from build123d import *

# Parameters (mm, degrees)
CORTAR_EXTRUIR1_DEPTH   = 9
CROQUIS5_R              = 4
CORTAR_EXTRUIR3_DEPTH   = 27
CROQUIS6_R              = 2
CORTAR_EXTRUIR4_DEPTH   = 10
CROQUIS7_R              = 2
SALIENTE_EXTRUIR1_DEPTH = 4.5
CROQUIS8_R              = 7
CROQUIS8_R_2            = 2
CORTAR_EXTRUIR5_DEPTH   = 4.5


with BuildPart() as part:
    # Croquis1 → Revolución1 (revolve)
    with BuildSketch(Plane(origin=(0, 0, 0), x_dir=(1, 0, 0), z_dir=(0, 1, 0))):
        Polygon((0, 1.5), (0, -9.5), (7, -9.5), (7, -13), (12.5, -13), (27.5, -13), (27.5, -7.5), (20, -7.5), (20, -2.5), (27.5, -2.5), (27.5, 2.5), (20, 2.5), (20, 7.5), (27.5, 7.5), (27.5, 13), (12.5, 13), (12.5, 6.5), (7.5, 1.5), align=None)
    revolve(axis=Axis((0, 0, 0), (0, 0, -1)))

    # Croquis2 → Cortar-Extruir1 (cut)
    with BuildSketch(Plane(origin=(0, 0, -1.5), x_dir=(-1, 0, 0), z_dir=(0, 0, -1))):
        Polygon((7.505553499, 0), (3.75277675, 6.5), (-3.75277675, 6.5), (-7.505553499, 0), (-3.75277675, -6.5), (3.75277675, -6.5), align=None)
    extrude(amount=-CORTAR_EXTRUIR1_DEPTH, mode=Mode.SUBTRACT)

    # Croquis5 → Cortar-Extruir3 (cut, through all)
    with BuildSketch(Plane.XY.offset(13)):
        with Locations((0, 24.5)):
            Circle(CROQUIS5_R)
        with Locations((12.25, 21.217622393)):
            Circle(CROQUIS5_R)
        with Locations((21.217622393, 12.25)):
            Circle(CROQUIS5_R)
        with Locations((24.5, 0)):
            Circle(CROQUIS5_R)
        with Locations((21.217622393, -12.25)):
            Circle(CROQUIS5_R)
        with Locations((12.25, -21.217622393)):
            Circle(CROQUIS5_R)
        with Locations((0, -24.5)):
            Circle(CROQUIS5_R)
        with Locations((-12.25, -21.217622393)):
            Circle(CROQUIS5_R)
        with Locations((-21.217622393, -12.25)):
            Circle(CROQUIS5_R)
        with Locations((-24.5, 0)):
            Circle(CROQUIS5_R)
        with Locations((-21.217622393, 12.25)):
            Circle(CROQUIS5_R)
        with Locations((-12.25, 21.217622393)):
            Circle(CROQUIS5_R)
    extrude(amount=-CORTAR_EXTRUIR3_DEPTH, mode=Mode.SUBTRACT)

    # Croquis6 → Cortar-Extruir4 (cut)
    with BuildSketch(Plane(origin=(0, 0, 7.5), x_dir=(-1, 0, 0), z_dir=(0, 0, -1))):
        Circle(CROQUIS6_R)
    extrude(amount=-CORTAR_EXTRUIR4_DEPTH, mode=Mode.SUBTRACT)

    # Croquis7 → Saliente-Extruir1 (add)
    with BuildSketch(Plane(origin=(0, 0, 7.5), x_dir=(-1, 0, 0), z_dir=(0, 0, -1))):
        Polygon((3.75277675, -6.5), (7.505553499, 0), (3.75277675, 6.5), (-3.75277675, 6.5), (-7.505553499, 0), (-3.75277675, -6.5), align=None)
        Circle(CROQUIS7_R, mode=Mode.SUBTRACT)
    extrude(amount=SALIENTE_EXTRUIR1_DEPTH)

    # Croquis8 → Cortar-Extruir5 (cut)
    with BuildSketch(Plane.XY.offset(9.5)):
        Circle(CROQUIS8_R)
        Circle(CROQUIS8_R_2, mode=Mode.SUBTRACT)
    extrude(amount=-CORTAR_EXTRUIR5_DEPTH, mode=Mode.SUBTRACT)


solid = part.part
Build history of the part. All positions in model axes, mm. A direction names the side the tool comes from. Coordinates: 2 decimals unless noted, no trailing zeros. Write each loop counter-clockwise with the first axis right and the second up, starting at its lowest first coordinate (ties: lowest second). Pieces come first, ordered by that corner, then holes.
(1) Cut at B-B on x = -14.5. List the corners of the cut face in (y, z), and give its area (3 significant figures).
(2) Mould opens along Y. For faces 1 (the cylindrical face through (7.177, -26.547, 10.212)), 2 (the cylindrical face through (-17.82, 10.14, 10.29)), 3 (the cylindrical face through (-19.49, 19.4, -0.04)) say: pulls with the +Y half, pulls with the -Y half, needs draft (parallel to the pull), parting line crosses it, or undercut.
(3) Pin check, flat tips, straight feed: pin 1 Ø4 at (x, z) = (20, -4) entering from +Y; pin 2 Ø1.5 at (y, z) = (-3, 5) entering from +X; pin 3 Ø3 at (y, z) = (5, -0.5) entering from +X. Stop position of each tip, or through.
(4) 3-axis set-ups, long thin cutter, end or side, ignore diameter. For faces 4 (the flat face through (14.3, -14.3, -7.5)), 5 (the cylindrical face through (17.82, -10.14, -10.21)): which of +Z, -Z, +X, -X, +Y, -Y reach the whole face in a straight line?
(5) Drill centre lines: line 1 (Z direction, x = 7, y = 25); line 2 (X direction, y = 11, z = -0.75); line 3 (Y direction, x = 0, z = 10). Where is each one in solid material? Low to high.
(6) Cut at C-C on y = 10.5. State how many separate pieces and enclosed holes the cut face has, and give its area (3 significant figures).
Working result:
1. outline: (-17.91, -13) - (17.91, -13) - (17.91, -7.5) - (13.77, -7.5) - (13.77, -2.5) - (17.91, -2.5) - (17.91, 2.5) - (13.77, 2.5) - (13.77, 7.5) - (17.91, 7.5) - (17.91, 13) - (-17.91, 13) - (-17.91, 7.5) - (-13.77, 7.5) - (-13.77, 2.5) - (-17.91, 2.5) - (-17.91, -2.5) - (-13.77, -2.5) - (-13.77, -7.5) - (-17.91, -7.5) - close
1. area: 849 mm2
2. face 1: pulls with the -Y half
2. face 2: undercut
2. face 3: pulls with the +Y half
3. pin 1: stops at y = 20.18
3. pin 2: stops at x = 19.87
3. pin 3: stops at x = 27.28
4. face 4: none
4. face 5: +Z, -Z
5. line 1: z = -13 to -7.5, -2.5 to 2.5, 7.5 to 13
5. line 2: x = -25.2 to -25.02, -17.42 to 17.42, 25.02 to 25.2
5. line 3: y = -20.5 to -7, 7 to 20.5
6. separate pieces: 7
6. enclosed holes: 0
6. area: 818 mm2
